Input: dimensioned drawing with shaded views. Units: mm. Origin: part minimum x, y, z. Round coordinates to 2 decimals unless told otherwise and drop trailing zeros. Order: outer loops, then holes, each group sorted by start corner. A loop starts at its lowest first (then second) coordinate and runs counter-clockwise, first axis right, second up. Notation, with made-up numbers: M 64,-30.5 L 95,-30.5 A24 cw 95,-16.5 Z; hole C -34.5,13.25 d2. An arc over 180 degrees is marked long. One line per question, with ' | ' between items.
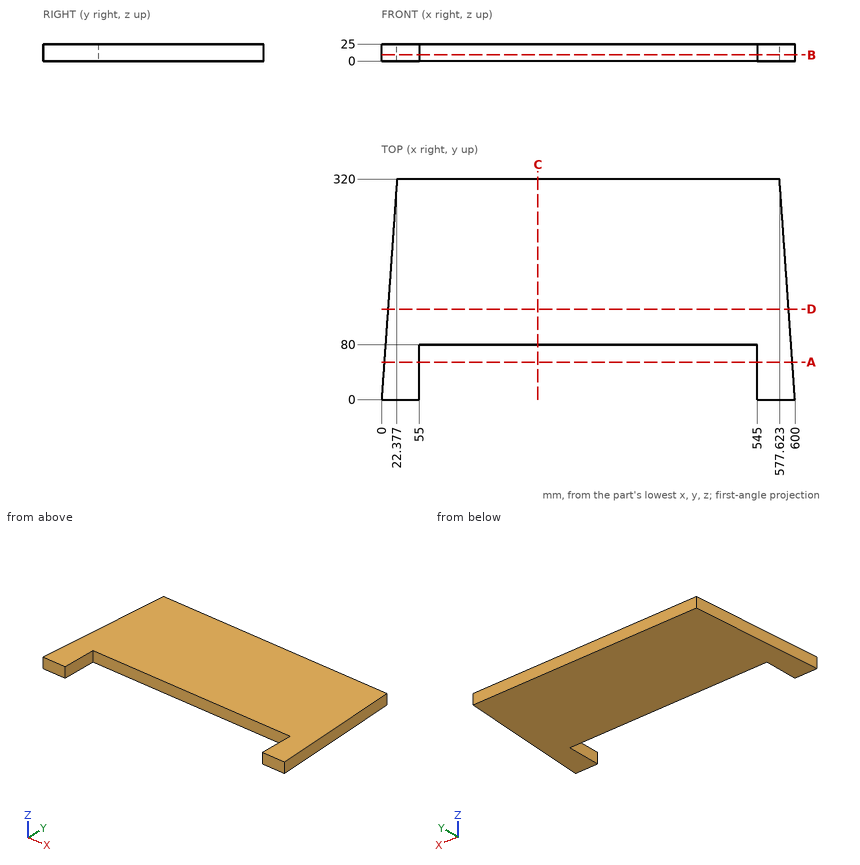
Item 1: First-contact query: pin 1 (1 mm diameter, centred on y = 213.5, z = 5, fed in from +X); pin 2 (5 mm diameter, centred on x = 202, z = 6.5, fed in from -Y); pin 3 (5 mm diameter, centred on y = 131.5, z = 4.5, fed in from -X); pin 4 (1 mm diameter, centred on x = 511.5, y = 279, fed in from -Z). Flat tips, straight axial feed; report the tip coordinate or a pass-through.
Report:
pin 1: x = 585.11 | pin 2: y = 80 | pin 3: x = 9.02 | pin 4: z = 0
Item 2: Section query D-D, the plane y = 131.5. Return loops of the section in (x, z) (1 decimal), plus the area to 3 significant figures.
Report:
outline: M 9.2,0 L 590.8,0 L 590.8,25 L 9.2,25 Z | area: 14,500 mm²
Item 3: Section query A-A, the plane y = 54.5. Return loops of the section in (x, z), plus the area to 3 significant figures.
Report:
outline: M 3.81,0 L 55,0 L 55,25 L 3.81,25 Z; M 545,0 L 596.19,0 L 596.19,25 L 545,25 Z | area: 2,560 mm²
Item 4: Section query B-B, the plane z = 9.25. Return loops of the section in (x, y).
Report:
outline: M 0,0 L 55,0 L 55,80 L 545,80 L 545,0 L 600,0 L 577.62,320 L 22.38,320 Z
Item 5: Section query C-C, the plane x = 227. Return loops of the section in (y, z), plus the area to 3 significant figures.
Report:
outline: M 80,0 L 320,0 L 320,25 L 80,25 Z | area: 6,000 mm²
Item 6: Line query: line 1 along Y through (x, z) = (144, 7.75); line 2 along X through (y, z) = (15, 5.25); line 3 along X through (y, z) = (289, 6.5). Output: solid intervals per line, ascending. Write a range as from..to.
Report:
line 1: 80..320 | line 2: 1.05..55, 545..598.95 | line 3: 20.21..579.79
